The model under review builds one solid part; all positions refer to its coordinate system, in mm. A direction names the side the tool comes from. Round coordinates to 2 decimals unless told otherwise and drop trailing zeros. Order: outer loops, then holes, each group sorted by start corner. A loop starts at its lowest first (then second) coordinate and runs counter-clockwise, first axis right, second up.
Autodesk Inventor part; units mm, degrees
ref_plane "YZ Plane" through (0, 0, 0) normal (1, 0, 0) x (0, 1, 0)
ref_plane "XZ Plane" through (0, 0, 0) normal (0, 1, 0) x (-1, 0, 0)
ref_plane "XY Plane" through (0, 0, 0) normal (0, 0, 1) x (1, 0, 0)
sketch "Sketch1" plane through (0, 0, 0) normal (0, 0, 1) x (1, 0, 0)
  line L0 (19.808, 75.5) -> (19.808, -72.5)
  line L1 (19.808, 75.5) -> (167.808, 75.5) construction
  line L2 (19.808, -72.5) -> (-60.192, -72.5)
  line L3 (-60.192, -72.5) -> (-60.192, -77.5)
  line L4 (-60.192, -72.5) -> (-55.192, -72.5) construction
  line L5 (-60.192, -77.5) -> (25.808, -77.5)
  line L6 (25.808, -77.5) -> (25.808, 80.5)
  line L7 (25.808, 80.5) -> (-59.192, 80.5)
  line L8 (-59.192, 80.5) -> (-59.192, 75.5)
  line L9 (-59.192, 75.5) -> (19.808, 75.5)
  point P0 (0, 0)
  dimension "d0" = 148
  dimension "d1" = 90
  dimension "d2" = 80
  dimension "d3" = 90
  dimension "d4" = 5
  dimension "d5" = 90
  dimension "d6" = 86
  dimension "d7" = 90
  dimension "d8" = 158
  dimension "d9" = 90
  dimension "d10" = 85
  dimension "d11" = 90
  dimension "d12" = 5
  dimension "d13" = 90
  dimension "d45" = 72.5
extrude "Extrusion1" add sketch "Sketch1" along normal mid plane 80
sketch "Sketch3" plane through (-59.192, 80.5, 40) normal (0, 1, 0) x (1, 0, 0)
  line L0 (60, 80) -> (0, 80)
  line L1 (30, 80) -> (30, 0) construction
  line L2 (60, 0) -> (0, 0)
  line L3 (30, 80) -> (120, 80) construction
  line L4 (85, 80) -> (85, 0)
  line L5 (85, 0) -> (0, 0)
  line L6 (0, 80) -> (85, 80)
  point P0 (59.817, 40)
  point P1 (15, 40)
  point P2 (30, 40)
  point P3 (30, 25)
  point P4 (45, 40)
  point P5 (30, 55)
  dimension "d30" = 90
  dimension "d31" = 55
  dimension "d32" = 40
  dimension "d33" = 15
  dimension "d36" = 360
hole "Hole2" at (-14.192, 80.5, 0) at (-29.192, 80.5, 15) at (-44.192, 80.5, 0) at (-29.192, 80.5, -15) direction (0, -1, 0) diameter 2.459 depth 5 counterbore diameter 6 counterbore depth 1
sketch "Sketch5" plane through (-60.192, -77.5, 40) normal (0, -1, 0) x (1, 0, 0)
  line L0 (31, -80) -> (31, 0) construction
  line L1 (31, -80) -> (111, -80) construction
  line L2 (86, -80) -> (86, 0)
  line L3 (0, 0) -> (86, 0)
  line L4 (86, -80) -> (0, -80)
  point P0 (60.192, -40)
  point P1 (31, -40)
  point P2 (16, -40)
  point P3 (31, -55)
  point P4 (46, -40)
  point P5 (31, -25)
  dimension "d48" = 90
  dimension "d49" = 55
  dimension "d50" = 15
  dimension "d53" = 360
hole "Hole3" at (-29.192, -77.5, 15) at (-29.192, -77.5, -15) at (-44.192, -77.5, 0) at (-14.192, -77.5, 0) direction (0, 1, 0) diameter 2.459 depth 5 counterbore diameter 6 counterbore depth 1
sketch "Sketch6" plane through (19.808, -72.5, 40) normal (-1, 0, 0) x (0, 0, 1)
  point P0 (-40, 72.5)
  point P1 (-40, 90.53)
  point P2 (-58.03, 72.5)
  point P3 (-40, 54.47)
  point P4 (-21.97, 72.5)
  dimension "d62" = 18.03
  dimension "d65" = 360
hole "Hole4" at (19.808, 0, -18.03) at (19.808, -18.03, 0) at (19.808, 0, 18.03) at (19.808, 18.03, 0) direction (1, 0, 0) diameter 4.134 end through all counterbore diameter 9.93 counterbore depth 3
properties part number "sidebracket"
(1) For faces 5 (the flat face through (-16, 80.5, -9)), 6 (the flat face through (-20, 75.5, -1)), 7 (the cylindrical face through (21.329, -1.491, 22.766)), 8 (the cylindrical face through (-11.263, 79.993, -0.65)), list the 3-axis set-ups (+Z, -Z, +X, -X, +Y, -Y) from which the entire face can be reached by the end or side of a thin tool; tool diameter is ignored.
Data:
face 5: +Z, -Z, +X, -X, +Y
face 6: +Z, -Z, -X
face 7: -X
face 8: +Y
(2) Consider section C-C (z = -29). Write out the cut boundary in (x, y).
Data:
outline: (-60.19, -77.5) - (25.81, -77.5) - (25.81, 80.5) - (-59.19, 80.5) - (-59.19, 75.5) - (19.81, 75.5) - (19.81, -72.5) - (-60.19, -72.5) - close
(3) Consider section B-B (y = -18.03). Write out the cut boundary in (x, z) (3 decimals).
Data:
outline: (19.808, -40) - (25.808, -40) - (25.808, -2.067) - (22.808, -2.067) - (22.808, -4.965) - (19.808, -4.965) - close; (19.808, 4.965) - (22.808, 4.965) - (22.808, 2.067) - (25.808, 2.067) - (25.808, 40) - (19.808, 40) - close
(4) To check wall thickness, follow probe 1 along Z at (x, y) = (24.45, 0); probe 2 along X at (y, z) = (-77.15, 0); probe 3 along Y at (x, z) = (-13.5, -9). State the ranges of each line that lie inside material, in increasing order.
Data:
probe 1: z = -40 to -20.1, -15.96 to 15.96, 20.1 to 40
probe 2: x = -60.19 to -47.19, -41.19 to -17.19, -11.19 to 25.81
probe 3: y = -77.5 to -72.5, 75.5 to 80.5
(5) Consider section D-D (y = 7). Write out the cut boundary in (x, z), and give its area (3 significant figures).
Data:
outline: (19.81, -40) - (25.81, -40) - (25.81, 40) - (19.81, 40) - close
area: 480 mm2
(6) Insertion check: pin 1 (5 mm diameter, centred on y = 20, z = -0.5, fed in from -X); pin 2 (4 mm diameter, centred on x = -29.192, z = -15, fed in from -Y); pin 3 (3 mm diameter, centred on y = -25, z = 13.5, fed in from -X). Each pin has a flat end and moves straight along its axis. Give the tip position at first contact, or say it passes through.
Data:
pin 1: stops at x = 22.81
pin 2: stops at y = -76.5
pin 3: stops at x = 19.81
(7) Draft analysis for pull direction X (two halves, no side actions). For faces 1 (the flat face through (19.808, 3, -1)), 2 (the flat face through (-18, -77.5, -1)), 3 (the cylindrical face through (-31.22, -76.99, 17.21)), 4 (the flat face through (-28.6, 79.5, 16.3)), state which applies: pulls with the +X half, pulls with the -X half, needs draft (parallel to the pull), parting line crosses it, or undercut.
Data:
face 1: pulls with the -X half
face 2: needs draft
face 3: undercut
face 4: undercut
(8) Consider section A-A (x = -34.5). Write out the cut boundary in (y, z).
Data:
outline: (-77.5, -40) - (-72.5, -40) - (-72.5, 40) - (-77.5, 40) - close; (75.5, -40) - (80.5, -40) - (80.5, 40) - (75.5, 40) - close
